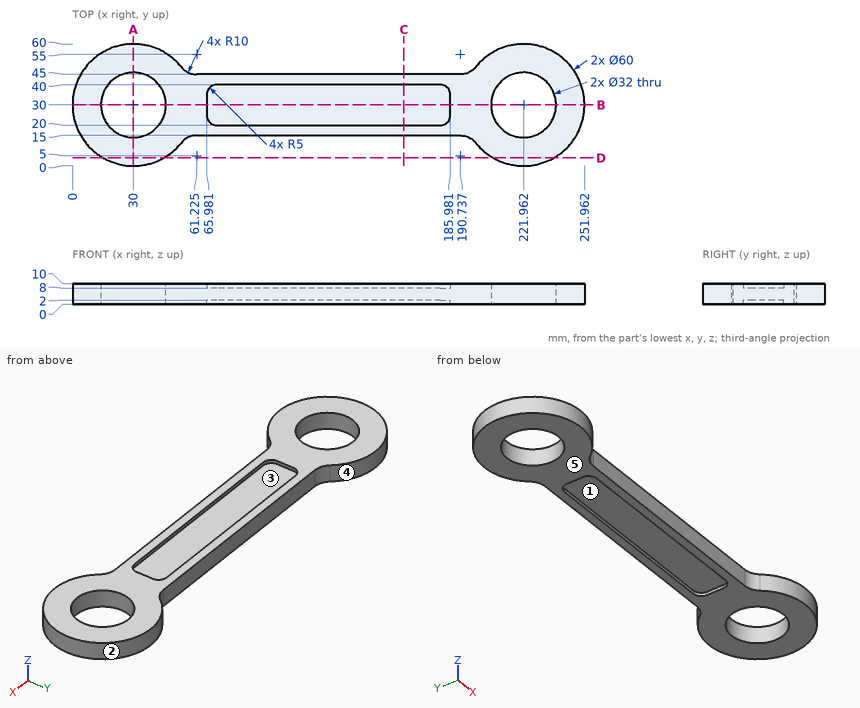
Here's the drawing with two shaded views (mm, measured from the low corner). I have some questions. A direction names the side the tool comes from. Coordinates: 2 decimals unless noted, no trailing zeros. Order: outer loops, then holes, each group sorted by start corner. A loop starts at its lowest first (then second) coordinate and runs counter-clockwise, first axis right, second up.
Q1. Please list where these lines run through material, in increasing order: L1, parallel to Y at x = 160.5, z = 8.5; L2, parallel to X at y = 15.5, z = 9.75 (1 decimal); L3, parallel to X at y = 18, z = 3.5 (1 decimal).
Q2. Suppose I cut it at A-A on x = 30. Please give me the cut outline in (y, z).
Q3. Suppose I cut it at C-C on x = 163. Please give me the cut outline in (y, z).
Q4. Suppose I cut it at B-B on y = 30. Please give me the cut outline in (x, z).
Q5. Thinking about a two-plate mould opening in Y: for the marked faces 3, 4 and 5, which applies, released by +Y, released by -Y, zero draft, split by the parting line, or undercut?
Q6. Will these pins go through, and if not, where does the flat tip stop? pin 1 (2 mm diameter, centred on y = 31.5, z = 9, fed in from +X); pin 2 (4 mm diameter, centred on y = 45, z = 8.5, fed in from +X); pin 3 (6 mm diameter, centred on x = 153.5, y = 29.5, fed in from +Z).
Q7. Which directions (+Z, -Z, +X, -X, +Y, -Y) give clear straight access to the entire face, cutting with the end or side of a thin tool? Please do the marked faces 1 and 2.
Q8. Suppose I cut it at D-D on y = 4. Please give me the cut outline in (x, z) (1 decimal).
Answer:
1. L1: y = 15 to 20, 40 to 45
1. L2: x = 3.7 to 23.2, 36.8 to 215.2, 228.7 to 248.2
1. L3: x = 2.5 to 19.4, 40.6 to 211.4, 232.5 to 249.5
2. outline: (0, 0) - (14, 0) - (14, 10) - (0, 10) - close; (46, 0) - (60, 0) - (60, 10) - (46, 10) - close
3. outline: (15, 0) - (20, 0) - (20, 2) - (40, 2) - (40, 0) - (45, 0) - (45, 10) - (40, 10) - (40, 8) - (20, 8) - (20, 10) - (15, 10) - close
4. outline: (0, 0) - (14, 0) - (14, 10) - (0, 10) - close; (46, 0) - (65.98, 0) - (65.98, 2) - (185.98, 2) - (185.98, 0) - (205.96, 0) - (205.96, 10) - (185.98, 10) - (185.98, 8) - (65.98, 8) - (65.98, 10) - (46, 10) - close; (237.96, 0) - (251.96, 0) - (251.96, 10) - (237.96, 10) - close
5. face 3: undercut
5. face 4: split by the parting line
5. face 5: zero draft
6. pin 1: stops at x = 251.96
6. pin 2: stops at x = 249
6. pin 3: stops at z = 8
7. face 1: -Z
7. face 2: +Z, -Z
8. outline: (15, 0) - (45, 0) - (45, 10) - (15, 10) - close; (207, 0) - (236.9, 0) - (236.9, 10) - (207, 10) - close
